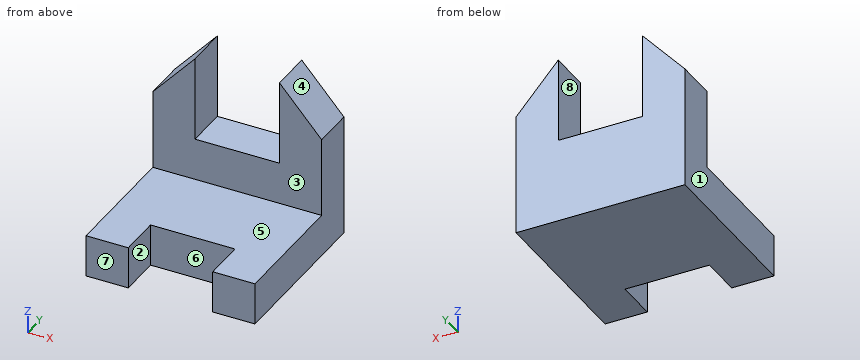
```python
from build123d import *

# Parameters (mm, degrees)
F1_DEPTH  = 25.4
F2_W      = 76.2
F2_H      = 25.4
F3_DEPTH  = 101.6
F4_W      = 50.8
F4_H      = 25.4
F5_DEPTH  = 25.4
F7_DEPTH  = 25.4
F9_DEPTH  = 25.4
F10_DEPTH = 25.4
F11_DEPTH = 25.4
F12_DEPTH = 25.4


with BuildPart() as f1:
    # F0 (on Front) → F1 (new body)
    with BuildSketch(Plane.XZ):
        Polygon((-101.6, 0), (0, 0), (0, 101.6), (-25.4, 101.6), (-25.4, 50.8), (-76.2, 50.8), (-76.2, 101.6), (-101.6, 101.6), align=None)
    extrude(amount=F1_DEPTH)

    # F2 (on Right) → F3 (join)
    with BuildSketch(Plane.YZ):
        with Locations((-38.1, 12.7)):
            Rectangle(F2_W, F2_H)
    extrude(amount=-F3_DEPTH)

    # F4 (on face) → F5 (cut)
    with BuildSketch(Plane.XZ.offset(76.2)):
        with Locations((-50.8, 12.7)):
            Rectangle(F4_W, F4_H)
    extrude(amount=-F5_DEPTH, mode=Mode.SUBTRACT)

    # F6 (on face) → F7 (cut)
    with BuildSketch(Plane.XZ.offset(25.4)):
        Polygon((0, 101.6), (-25.4, 101.6), (0, 73.2019366858), align=None)
    extrude(amount=-F7_DEPTH, mode=Mode.SUBTRACT)

    # F8 (on face) → F9 (cut)
    with BuildSketch(Plane.XZ.offset(25.4)):
        Polygon((-101.6, 73.2019366858), (-76.2, 101.6), (-101.6, 101.6), align=None)
    extrude(amount=-F9_DEPTH, mode=Mode.SUBTRACT)

    # F10 (add): a face of the model
    f10_faces = [f1.faces().sort_by_distance(p)[0] for p in [
        (-12.7, -76.2, 12.7),
    ]]
    extrude(f10_faces, amount=F10_DEPTH)

    # F11 (add): a face of the model
    f11_faces = [f1.faces().sort_by_distance(p)[0] for p in [
        (-88.9, -76.2, 12.7),
    ]]
    extrude(f11_faces, amount=F11_DEPTH)

    # F12 (add): a face of the model
    f12_faces = [f1.faces().sort_by_distance(p)[0] for p in [
        (-50.8, -50.8, 12.7),
    ]]
    extrude(f12_faces, amount=F12_DEPTH)


solid = f1.part
```
Check sheet for the modelled part. Datum: model origin and axes. Units: mm. Face numbers are marked on the shaded views. A direction names the side the tool comes from. Coordinates: 2 decimals unless noted, no trailing zeros. Write each loop counter-clockwise with the first axis right and the second up, starting at its lowest first coordinate (ties: lowest second). Pieces come first, ordered by that corner, then holes. Notation, with made-up numbers: M 4.5,31 L 15.5,31 A19 ccw 15.5,53 Z; hole C 33.25,-3 d1. An arc over 180 degrees is marked long. Use one line per item in the form item = value.
Item 1: Gauge pin test, flat ends, axial feed: pin 1 Ø23 at (x, y) = (-52, -64.5) entering from +Z; pin 2 Ø2 at (x, y) = (-77.5, -12.5) entering from +Z; pin 3 Ø12.5 at (y, z) = (-17.5, 86.5) entering from +X. Record the tip position at first contact, or that the pin passes through.
Answer below:
pin_1 = 25.4
pin_2 = 101.26
pin_3 = -6.3
Item 2: Sectioned sample at B-B, the plane y = -94. Record the cut outline in (x, z), and give its area (3 significant figures).
Answer below:
outline = M -101.6,0 L -76.2,0 L -76.2,25.4 L -101.6,25.4 Z; M -25.4,0 L 0,0 L 0,25.4 L -25.4,25.4 Z
area = 1,290 mm^2
Item 3: Sectioned sample at A-A, the plane z = 59. Record the cut outline in (x, y).
Answer below:
outline = M -101.6,-25.4 L -76.2,-25.4 L -76.2,0 L -101.6,0 Z; M -25.4,-25.4 L 0,-25.4 L 0,0 L -25.4,0 Z
Item 4: Material ranges on L1, parallel to X at y = -15.5, z = 56.5; L2, parallel to Y at x = -80.5, z = 85; L3, parallel to X at y = -19.5, z = 82, recorded low to high. Write a range as from..to.
Answer below:
L1 = -101.6..-76.2, -25.4..0
L2 = -25.4..0
L3 = -93.73..-76.2, -25.4..-7.87
Item 5: Sectioned sample at D-D, the plane y = -9. Record the cut outline in (x, z), and give its area (3 significant figures).
Answer below:
outline = M -101.6,0 L 0,0 L 0,73.2 L -25.4,101.6 L -25.4,50.8 L -76.2,50.8 L -76.2,101.6 L -101.6,73.2 Z
area = 7,020 mm^2
Item 6: Sectioned sample at C-C, the plane x = -30. Record the cut outline in (y, z).
Answer below:
outline = M -76.2,0 L 0,0 L 0,50.8 L -25.4,50.8 L -25.4,25.4 L -76.2,25.4 Z
Item 7: Release check for a two-part mould opening along X. For the marked faces 1, 2 and 3 record: pulls with the +X half, pulls with the -X half, needs draft (parallel to the pull), parting line crosses it, or undercut.
Answer below:
face_1 = pulls with the -X half
face_2 = undercut
face_3 = needs draft
Item 8: Set-up check for the marked faces 4, 5, 6, 7 and 8: record each of +Z, -Z, +X, -X, +Y, -Y from which the full face is reachable in a straight line by a thin tool's end or side.
Answer below:
face_4 = +Z, +X, +Y, -Y
face_5 = +Z, +X, -X, -Y
face_6 = +Z, -Z, -Y
face_7 = +Z, -Z, +X, -X, -Y
face_8 = +Z, +Y, -Y
